For this review, use the dimensioned drawing (mm, ordinates from the lowest corner) and the shaded views. Coordinates: 2 decimals unless noted, no trailing zeros. Loops run counter-clockwise (first coordinate to the right, second up) from the corner with the lowest first, then second, coordinate; pieces in that order, holes last.
1. Clearance check with flat-ended pins moving along their axes: P1, Ø6, axis at x = 32, z = 21.5, coming from the -Y side; P2, Ø1.5, axis at x = 6, y = 2, coming from the -Z side (1 decimal). State where each tip first meets the part, or that it passes through.
2. Take a section at B-B, the plane x = 20.32. State the section outline as (y, z) points.
3. To check wall thickness, follow probe 1 along Z at (x, y) = (20.32, 1.95); probe 2 along Y at (x, z) = (33.5, 21); probe 3 along Z at (x, y) = (35.5, 0.8) (1 decimal). State the ranges of each line that lie inside material, in increasing order.
4. Mouldability with a two-part tool opening along Z and no side actions: class the marked faces 1 and 2 as pulls with the +Z half, pulls with the -Z half, needs draft (parallel to the pull), parting line crosses it, or undercut.
5. Take a section at A-A, the plane z = 20.32. State the section outline as (x, y) points.
6. Take a section at D-D, the plane z = 10.5. State the section outline as (x, y) points.
7. Take a section at C-C, the plane x = 32. State the section outline as (y, z) points.
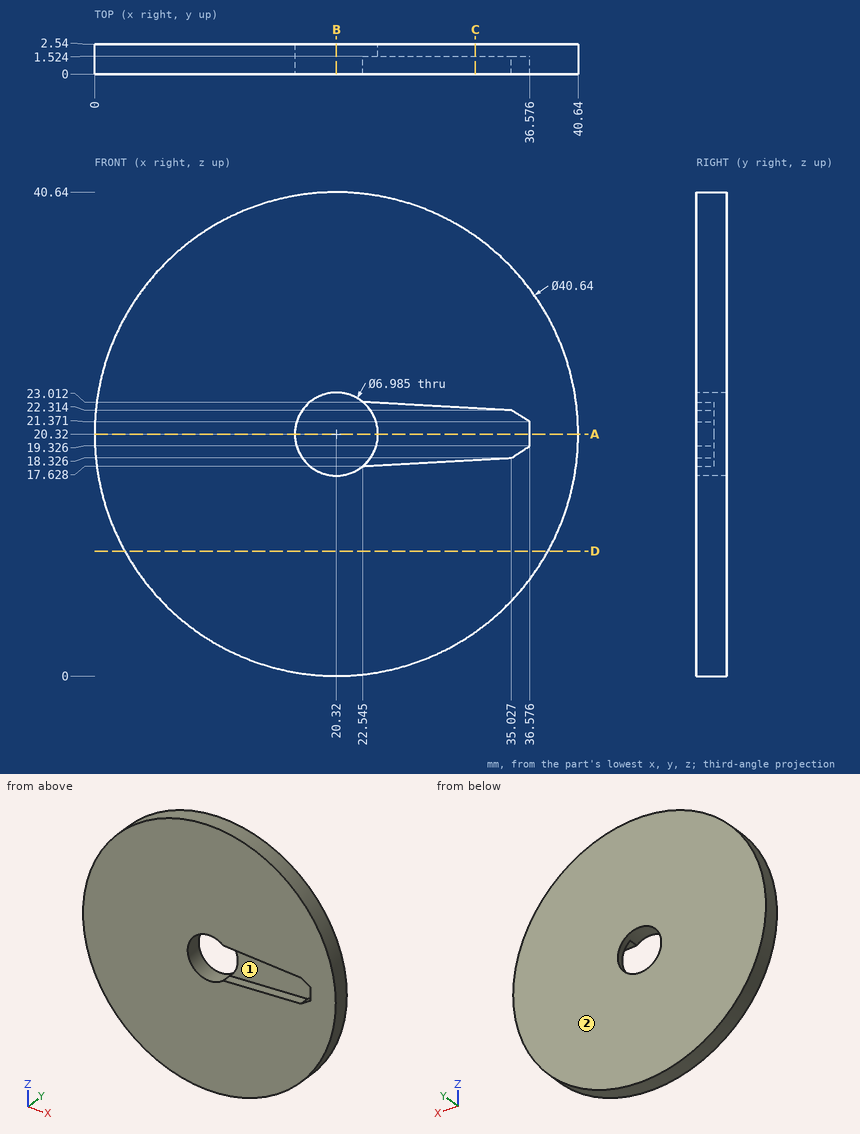
Results list:
1. P1: stops at y = 0
1. P2: stops at z = 5.2
2. outline: (0, 0) - (2.54, 0) - (2.54, 16.83) - (0, 16.83) - close; (0, 23.81) - (2.54, 23.81) - (2.54, 40.64) - (0, 40.64) - close
3. probe 1: z = 0 to 16.83, 23.81 to 40.64
3. probe 2: y = 1.52 to 2.54
3. probe 3: z = 6.8 to 18.6, 22 to 33.8
4. face 1: undercut
4. face 2: needs draft
5. outline: (0, 0) - (16.83, 0) - (16.83, 2.54) - (0, 2.54) - close; (23.81, 1.52) - (36.58, 1.52) - (36.58, 0) - (40.64, 0) - (40.64, 2.54) - (23.81, 2.54) - close
6. outline: (2.53, 0) - (38.11, 0) - (38.11, 2.54) - (2.53, 2.54) - close
7. outline: (0, 3.69) - (2.54, 3.69) - (2.54, 36.95) - (0, 36.95) - (0, 22.48) - (1.52, 22.48) - (1.52, 18.16) - (0, 18.16) - close
